The model under review builds one solid part; all positions refer to its coordinate system, in mm. A direction names the side the tool comes from. Give positions to 0.01 mm unless a question says otherwise; leave off trailing zeros. Use one line per item in the form item = value.
```python
from build123d import *


with BuildPart() as f1:
    # F0 (on Front) → F1 (revolve)
    with BuildSketch(Plane.XZ):
        with BuildLine():
            Line((31.75, 17.7578248391), (31.75, 21.5678248391))
            Line((31.75, 21.5678248391), (13.9625025913, 21.5678248391))
            Line((13.9625025913, 21.5678248391), (13.9625025913, 26.6478248391))
            Line((13.9625025913, 26.6478248391), (31.75, 26.6478248391))
            Line((31.75, 26.6478248391), (31.75, 34.2678248391))
            Line((31.75, 34.2678248391), (7.62, 34.2678248391))
            add(Edge.make_bspline(
                [(7.62, 50.8), (8.7946373317, 48.2662832015), (10.5938172445, 45.6910384811), (3.9703337235, 41.1560327641), (10.6575661956, 38.0275243968), (7.62, 34.2678248391)],
                knots=[0, 0, 0, 0, 0.3247209532, 0.6256741659, 1, 1, 1, 1], degree=3))
            Line((7.62, 50.8), (0, 50.8))
            Line((0, 50.8), (0, 0))
            ThreePointArc((0, 0), (16.8455899513, 4.7645191049), (31.75, 13.9478248391))
            Line((31.75, 13.9478248391), (31.75, 15.2178248391))
            Line((31.75, 15.2178248391), (13.9625025913, 15.2178248391))
            Line((13.9625025913, 15.2178248391), (13.9625025913, 17.7578248391))
            Line((13.9625025913, 17.7578248391), (31.75, 17.7578248391))
        make_face()
    revolve(axis=Axis((0, 0, 25.4), (0, 0, 1)))


solid = f1.part
```
1. The part is to be moulded in two halves that separate along Z. For faces 3 (the face through (13.32, 4.19, 24.14)), 4 (the face through (-6.883, -30.995, 30.511)), 5 (the face through (0, 0, 50.8)), say which applies: +Z half, -Z half, draft (parallel to the pull), parting line (faces both ways), or undercut.
Values:
face_3 = undercut
face_4 = draft
face_5 = +Z half
2. Tool access review of faces 1 (the face through (-6.883, -30.995, 19.689)), 2 (the face through (14, -7, 21.568)): name each direction out of +Z, -Z, +X, -X, +Y, -Y from which nothing blocks a thin tool from reaching the whole face with its end or side.
Values:
face_1 = +Z, -Z
face_2 = none
3. For L1, parallel to Z at x = 16.5, y = -22.5; L2, parallel to Z at x = -21.5, y = -20.5; L3, parallel to X at y = 11.5, z = 8.5, list the stretches that pass through material, from the lowest coordinate up.
Values:
L1 = 11.01 to 15.22, 17.76 to 21.57, 26.65 to 34.27
L2 = 12.33 to 15.22, 17.76 to 21.57, 26.65 to 34.27
L3 = -21.13 to 21.13
4. Add section A-A on y = 16. Count the separate pieces of the cut face and the enclosed holes in it, then the cut area to 3 significant figures.
Values:
separate_pieces = 3
enclosed_holes = 0
area = 1,050 mm^2
5. For pin 1 Ø8 at (x, y) = (-10.5, 17) entering from -Z; pin 2 Ø5 at (y, z) = (-2, 28) entering from -X; pin 3 Ø4 at (x, z) = (-12.5, 13.5) entering from -Y; pin 4 Ø5 at (x, z) = (-19.5, 19.5) entering from -Y, all flat-tipped, find the tip position at first contact; note any pin that passes through.
Values:
pin_1 = 4.39
pin_2 = -31.75
pin_3 = -29.95
pin_4 = -26.82
